Autodesk Inventor part; units mm, degrees
ref_plane "YZ Plane" through (0, 0, 0) normal (1, 0, 0) x (0, 1, 0)
ref_plane "XZ Plane" through (0, 0, 0) normal (0, 1, 0) x (-1, 0, 0)
ref_plane "XY Plane" through (0, 0, 0) normal (0, 0, 1) x (1, 0, 0)
sketch "Sketch1" plane through (0, 0, 0) normal (0, 1, 0) x (-1, 0, 0)
  line L0 (56.2338, 50.9905) -> (-39.0162, 50.9905)
  line L1 (-39.0162, 50.9905) -> (-39.0162, -88.7095)
  line L2 (-39.0162, -88.7095) -> (56.2338, -88.7095)
  line L3 (56.2338, -88.7095) -> (56.2338, 50.9905)
  point P0 (0, 0)
  dimension "d0" = 139.7
  dimension "d1" = 95.25
extrude "Extrusion1" add sketch "Sketch1" along normal blind 5.08
sketch "Sketch2" plane through (0, 5.08, 0) normal (0, 1, 0) x (1, 0, 0)
  line L0 (-56.2338, -50.9905) -> (39.0162, -50.9905)
  line L1 (39.0162, 88.7095) -> (-56.2338, 88.7095)
  line L2 (-56.2338, 88.7095) -> (-56.2338, -50.9905)
  point P0 (0, 0)
  point P1 (-43.5338, -44.6405)
  point P2 (13.6162, -44.6405)
  point P3 (13.6162, 82.3595)
  point P4 (-43.5338, 82.3595)
  dimension "d4" = 0
  dimension "d5" = 6.35
  dimension "d6" = 0
  dimension "d7" = 6.35
  dimension "d8" = 0
  dimension "d9" = 0
  dimension "d10" = 12.7
  dimension "d11" = 57.15
hole "Hole1" at (-43.5338, 5.08, 44.6405) at (13.6162, 5.08, 44.6405) at (13.6162, 5.08, -82.3595) at (-43.5338, 5.08, -82.3595) direction (0, -1, 0) diameter 4.4958 end through all
sketch "Sketch4" plane through (0, 5.08, 0) normal (0, 1, 0) x (1, 0, 0)
  circle A0 centre (-30.8338, 18.8595) radius 19.8293
  line L0 (-56.2338, -50.9905) -> (39.0162, -50.9905)
  line L1 (-56.2338, 88.7095) -> (-56.2338, -50.9905)
  point P0 (0, 0)
  dimension "d26" = 69.85
  dimension "d27" = 25.4
extrude "Extrusion3" add sketch "Sketch4" along normal blind 6.35
sketch "Sketch5" plane through (-30.8338, 11.43, -18.8595) normal (0, 1, 0) x (1, 0, 0)
  circle A0 centre (0, 0) radius 2.3813
  point P0 (30.8338, -18.8595)
  dimension "d30" = 4.7625
extrude "Extrusion4" cut sketch "Sketch5" against normal blind 33.3375
sketch "Sketch6" plane through (0, 0, 0) normal (0, -1, 0) x (1, 0, 0)
  circle A0 centre (-30.8338, -18.8595) radius 2.3813
  circle A1 centre (-30.8338, -18.8595) radius 9.525
  point P0 (0, 0)
  dimension "d33" = 19.05
extrude "Extrusion5" cut sketch "Sketch6" against normal blind 5.08
properties part number "Slider"
Geometry check sheet. Reference: the model listing, model coordinates, mm. A direction names the side the tool comes from. Round coordinates to 2 decimals unless told otherwise and drop trailing zeros. Order: outer loops, then holes, each group sorted by start corner. A loop starts at its lowest first (then second) coordinate and runs counter-clockwise, first axis right, second up. Notation, with made-up numbers: M 89,16.25 L 135,16.25 A33 ccw 135,49.25 Z; hole C 71,-18 d11. An arc over 180 degrees is marked long. Answer as CSV lines item,"result".
1) Sectioned sample at D-D on x = -49. Record the cut outline in (y, z).
Entries:
outline,"M 0,-88.71 L 5.08,-88.71 L 5.08,-26.81 L 11.43,-26.81 L 11.43,-10.91 L 5.08,-10.91 L 5.08,50.99 L 0,50.99 Z"
2) Sectioned sample at C-C on z = 37.5. Record the cut outline in (x, y).
Entries:
outline,"M -56.23,0 L 39.02,0 L 39.02,5.08 L -56.23,5.08 Z"
3) Tool access check on faces 1 (the face through (15.81, 2.5, 44.15)), 2 (the face through (-12.517, 8.211, -26.454)), 3 (the face through (-29, 5.08, -21)). Record the directions out of +Z, -Z, +X, -X, +Y, -Y that give a thin tool (end or side, any length) a straight path to the whole face; none if there is none.
Entries:
face 1,"+Y, -Y"
face 2,"+Y"
face 3,"-Y"
4) Sectioned sample at A-A on x = -26.5. Record the cut outline in (y, z).
Entries:
outline,"M 0,-88.71 L 5.08,-88.71 L 5.08,-38.21 L 11.43,-38.21 L 11.43,0.49 L 5.08,0.49 L 5.08,50.99 L 0,50.99 L 0,-10.38 L 5.08,-10.38 L 5.08,-27.34 L 0,-27.34 Z"
5) Gauge pin test, flat end, axial feed: pin 1 Ø6 at (x, z) = (13.62, 44.64) entering from +Y. Record the tip position at first contact, or that the pin passes through.
Entries:
pin 1,"y = 5.08"
6) Thickness scan on probe 1 along Z at (x, y) = (12.5, 5); probe 2 along Z at (x, y) = (15.5, 2.5); probe 3 along Y at (x, z) = (28, -62). Record the ranges inside material, lowest first. Write a range as [from, to].
Entries:
probe 1,"[-88.71, -84.31], [-80.41, 42.69], [46.59, 50.99]"
probe 2,"[-88.71, -83.59], [-81.13, 43.41], [45.87, 50.99]"
probe 3,"[0, 5.08]"
7) Mould release check, pull along Z, two halves, no side actions. Record for faces 4 (the face through (-8, 0, -18)), 5 (the face through (-32.724, 8.299, -17.411)), 6 (the face through (-9, 3, 50.99)): +Z half, -Z half, draft (parallel to the pull), parting line (faces both ways), or undercut.
Entries:
face 4,"draft"
face 5,"undercut"
face 6,"+Z half"
8) Sectioned sample at B-B on y = 3.5. Give the number of separate pieces and of enclosed holes in the cut face, and give its area (3 significant figures).
Entries:
separate pieces,"1"
enclosed holes,"5"
area,"13,000 mm2"
